```python
from build123d import *

# Parameters (mm, degrees)
SKETCH1_W           = 310
SKETCH1_H           = 310
BOSS_EXTRUDE1_DEPTH = 6
BOSS_EXTRUDE2_DEPTH = 6
SKETCH4_R           = 51.5
CUT_EXTRUDE1_DEPTH  = 439.570404838
SKETCH11_R          = 2
CUT_EXTRUDE5_DEPTH  = 439.570404838
SKETCH12_W          = 25
SKETCH12_H          = 10
BOSS_EXTRUDE3_DEPTH = 6.5
SKETCH13_W          = 25
SKETCH13_H          = 112
BOSS_EXTRUDE4_DEPTH = 8


with BuildPart() as part:
    # Sketch1 → Boss-Extrude1 (new body)
    with BuildSketch(Plane.XY):
        with Locations((155, -155)):
            Rectangle(SKETCH1_W, SKETCH1_H)
    extrude(amount=BOSS_EXTRUDE1_DEPTH)

    # Sketch3 → Boss-Extrude2 (add)
    with BuildSketch(Plane.XY.offset(6)):
        Polygon((302, -8), (302, -33), (302, -277), (302, -302), (277, -302), (33, -302), (8, -302), (8, -277), (8, -33), (8, -8), (33, -8), (277, -8), align=None)
        Polygon((268.286796564, -20.5), (223.286796564, -65.5), (86.713203436, -65.5), (41.713203436, -20.5), align=None, mode=Mode.SUBTRACT)
        Polygon((20.5, -41.713203436), (65.5, -86.713203436), (65.5, -223.286796564), (20.5, -268.286796564), align=None, mode=Mode.SUBTRACT)
        Polygon((41.713203436, -289.5), (86.713203436, -244.5), (223.286796564, -244.5), (268.286796564, -289.5), align=None, mode=Mode.SUBTRACT)
        Polygon((289.5, -41.713203436), (244.5, -86.713203436), (244.5, -223.286796564), (289.5, -268.286796564), align=None, mode=Mode.SUBTRACT)
    extrude(amount=BOSS_EXTRUDE2_DEPTH)

    # Sketch4 → Cut-Extrude1 (cut, through all)
    with BuildSketch(Plane.XY.offset(12)):
        with Locations((155, -155)):
            Circle(SKETCH4_R)
    extrude(amount=-CUT_EXTRUDE1_DEPTH, mode=Mode.SUBTRACT)

    # Sketch11 → Cut-Extrude5 (cut, through all)
    with BuildSketch(Plane(origin=(0, 0, 0), x_dir=(-1, 0, 0), z_dir=(0, 0, -1))):
        with Locations((-55, -55)):
            Circle(SKETCH11_R)
        with Locations((-55, -255)):
            Circle(SKETCH11_R)
    extrude(amount=-CUT_EXTRUDE5_DEPTH, mode=Mode.SUBTRACT)

    # Sketch12 → Boss-Extrude3 (add)
    with BuildSketch(Plane(origin=(0, 0, 0), x_dir=(-1, 0, 0), z_dir=(0, 0, -1))):
        with Locations((-272.5, -104)):
            Rectangle(SKETCH12_W, SKETCH12_H)
        with Locations((-272.5, -206)):
            Rectangle(SKETCH12_W, SKETCH12_H)
    extrude(amount=BOSS_EXTRUDE3_DEPTH)

    # Sketch13 → Boss-Extrude4 (add)
    with BuildSketch(Plane(origin=(0, 0, -6.5), x_dir=(-1, 0, 0), z_dir=(0, 0, -1))):
        with Locations((-272.5, -155)):
            Rectangle(SKETCH13_W, SKETCH13_H)
    extrude(amount=BOSS_EXTRUDE4_DEPTH)


solid = part.part
```
Work out the finished part from the listing and answer in its coordinate system (mm). A direction names the side the tool comes from. Give positions to 0.01 mm unless a question says otherwise; leave off trailing zeros. Loops run counter-clockwise (first coordinate to the right, second up) from the corner with the lowest first, then second, coordinate; pieces in that order, holes last. Notation, with made-up numbers: (65, 78) -> (81, 78) arc R23 cw to (81, 93) -> close; hole circle Ø4 at (0, -34). An arc over 180 degrees is marked (long way). Use CSV: the item, a comma, the result in double quotes.
1. The mould has two halves that part along Z. Classify faces 1 (the flat face through (273, -154, -6.5)), 2 (the flat face through (43, -153, 6)), 3 (the flat face through (64.528, -43.315, 8.958)): +Z half, -Z half, draft (parallel to the pull), parting line (faces both ways), or undercut.
Found:
face 1,"undercut"
face 2,"+Z half"
face 3,"draft"
2. A tool of negligible diameter and unlimited length cuts with its end or side. For faces 4 (the flat face through (260, -156, -9)), 5 (the flat face through (273, -211, -7)), 6 (the flat face through (267.315, -63.898, 8.958)), 7 (the flat face through (273, -99, -7)), from which of +Z, -Z, +X, -X, +Y, -Y can it reach the whole face along a straight path? Write none if from no direction.
Found:
face 4,"-Z, -X, +Y, -Y"
face 5,"-Z, +X, -X, -Y"
face 6,"+Z"
face 7,"-Z, +X, -X, +Y"
3. The part is cut by section C-C (x = 264). Write down the section's boundary in (y, z).
Found:
outline,"(-310, 0) -> (-211, 0) -> (-211, -14.5) -> (-99, -14.5) -> (-99, 0) -> (0, 0) -> (0, 6) -> (-8, 6) -> (-8, 12) -> (-20.5, 12) -> (-20.5, 6) -> (-24.79, 6) -> (-24.79, 12) -> (-67.21, 12) -> (-67.21, 6) -> (-242.79, 6) -> (-242.79, 12) -> (-285.21, 12) -> (-285.21, 6) -> (-289.5, 6) -> (-289.5, 12) -> (-302, 12) -> (-302, 6) -> (-310, 6) -> close; hole (-201, -6.5) -> (-109, -6.5) -> (-109, 0) -> (-201, 0) -> close"
4. The part is cut by section D-D (x = 35). Write down the section's boundary in (y, z).
Found:
outline,"(-310, 0) -> (0, 0) -> (0, 6) -> (-8, 6) -> (-8, 12) -> (-56.21, 12) -> (-56.21, 6) -> (-253.79, 6) -> (-253.79, 12) -> (-302, 12) -> (-302, 6) -> (-310, 6) -> close"
5. Straight lines are drawn through the part: line 1 (Y direction, x = 55, z = 5.25); line 2 (X direction, y = -188.5, z = 6.25); line 3 (Z direction, x = 175, y = -282). For each, find the intervals that lie inside material, in ascending order.
Found:
line 1,"-310 to -257, -253 to -57, -53 to 0"
line 2,"8 to 20.5, 65.5 to 115.88, 194.12 to 244.5, 289.5 to 302"
line 3,"0 to 6"
6. The part is cut by section A-A (x = 155). Write down the section's boundary in (y, z), then the cut area to 3 significant figures.
Found:
outline,"(-310, 0) -> (-206.5, 0) -> (-206.5, 12) -> (-244.5, 12) -> (-244.5, 6) -> (-289.5, 6) -> (-289.5, 12) -> (-302, 12) -> (-302, 6) -> (-310, 6) -> close; (-103.5, 0) -> (0, 0) -> (0, 6) -> (-8, 6) -> (-8, 12) -> (-20.5, 12) -> (-20.5, 6) -> (-65.5, 6) -> (-65.5, 12) -> (-103.5, 12) -> close"
area,"1,850 mm^2"
7. The part is cut by section B-B (y = -155). Write down the section's boundary in (x, z).
Found:
outline,"(0, 0) -> (103.5, 0) -> (103.5, 12) -> (65.5, 12) -> (65.5, 6) -> (20.5, 6) -> (20.5, 12) -> (8, 12) -> (8, 6) -> (0, 6) -> close; (206.5, 0) -> (310, 0) -> (310, 6) -> (302, 6) -> (302, 12) -> (289.5, 12) -> (289.5, 6) -> (244.5, 6) -> (244.5, 12) -> (206.5, 12) -> close; (260, -14.5) -> (285, -14.5) -> (285, -6.5) -> (260, -6.5) -> close"
8. Flat-ended cylindrical pins translate along their axes: pin 1 Ø2 at (y, z) = (-241.5, -2.5) entering from -X; pin 2 Ø6.5 at (y, z) = (-111.5, 9.5) entering from -X; pin 3 Ø3 at (x, z) = (226.5, 10) entering from -Y; pin 4 Ø5 at (y, z) = (-147, 10) entering from +X. Find the tip coordinate at first contact, or state that the pin passes through.
Found:
pin 1,"through"
pin 2,"x = 8"
pin 3,"y = -302"
pin 4,"x = 302"
